Read the model definition and answer for the solid it produces. Units are mm, in the model's axes. Face numbers are marked on the shaded views. Give positions to 0.01 mm unless a question says otherwise; leave off trailing zeros. Order: outer loops, then holes, each group sorted by start corner. A loop starts at its lowest first (then second) coordinate and runs counter-clockwise, first axis right, second up. Notation, with made-up numbers: (72.25, 37.25) - (87.25, 37.25) arc R30 ccw to (87.25, 73.25) - close; hole circle Ø5 at (59.5, 42). An arc over 180 degrees is marked (long way). Use a Markdown table: item, result. Add a question column.
1. A flat-ended cylindrical pin translates along its axis: P1, Ø1, axis at x = -5.5, z = 0.5, coming from the +Y side. Find the tip coordinate at first contact, or state that the pin passes through.
2. For a pull along Y with two mould halves and no side action, classify the marked faces 1 and 2 as released by +Y, released by -Y, zero draft, split by the parting line, or undercut.
3. Consider L1, parallel to Y at x = 0, z = 0.6; L2, parallel to Y at x = 2, z = 1.1; L3, parallel to X at y = 13.5, z = 2.1. Determine where each line is inside the solid, lowest interval first.
4. A cutting plane is placed at A-A on x = 0. Determine the outline of the cut face in (y, z), and give its area (3 significant figures).
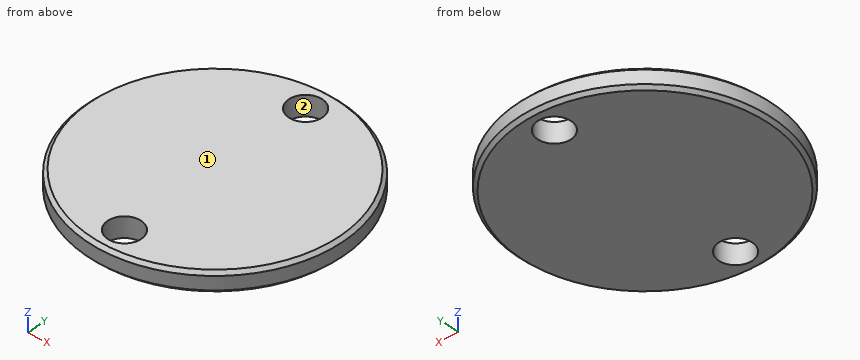
```python
from build123d import *

# Parameters (mm, degrees)
SKETCH_1_R          = 19
EXTRUDE_1_DEPTH     = 3
SKETCH_2_R          = 2.5
CUT_EXTRUDE_1_DEPTH = 13
CHAMFER_1_SIZE      = 0.5


with BuildPart() as part:
    # 草图1 → 拉伸1 (new body)
    with BuildSketch(Plane.XY):
        Circle(SKETCH_1_R)
    extrude(amount=EXTRUDE_1_DEPTH)

    # 草图2 → 切除-拉伸1 (cut)
    with BuildSketch(Plane.XY.offset(3)):
        with Locations((0, 15)):
            Circle(SKETCH_2_R)
        with Locations((0, -15)):
            Circle(SKETCH_2_R)
    extrude(amount=-CUT_EXTRUDE_1_DEPTH, mode=Mode.SUBTRACT)

    # 倒角1
    chamfer_1_edges = [part.edges().sort_by_distance(p)[0] for p in [
        (-19, 0, 0),
        (-19, 0, 3),
    ]]
    chamfer(chamfer_1_edges, length=CHAMFER_1_SIZE)


solid = part.part
```
Output values:
| question | item | result |
|---|---|---|
| 1 | P1 | y = 18.33 |
| 2 | face 1 | zero draft |
| 2 | face 2 | undercut |
| 3 | L1 | -19 to -17.5, -12.5 to 12.5, 17.5 to 19 |
| 3 | L2 | -18.89 to -16.5, -13.5 to 13.5, 16.5 to 18.89 |
| 3 | L3 | -13.37 to -2, 2 to 13.37 |
| 4 | outline | (-19, 0.5) - (-18.5, 0) - (-17.5, 0) - (-17.5, 3) - (-18.5, 3) - (-19, 2.5) - close; (-12.5, 0) - (12.5, 0) - (12.5, 3) - (-12.5, 3) - close; (17.5, 0) - (18.5, 0) - (19, 0.5) - (19, 2.5) - (18.5, 3) - (17.5, 3) - close |
| 4 | area | 83.5 mm² |
